Autodesk Inventor part; units mm, degrees
ref_plane "Work Plane1" through (99.0561, 66.015, -1.0424) normal (0, 1, 0) x (-0.9985, 0, 0.0543)
ref_plane "YZ Plane" through (0, 0, 0) normal (1, 0, 0) x (0, 1, 0)
ref_plane "XZ Plane" through (0, 0, 0) normal (0, 1, 0) x (-1, 0, 0)
ref_plane "Work Plane1" through (99.0561, 66.015, -1.0424) normal (0, 1, 0) x (-0.9985, 0, 0.0543)
sketch "Sketch1" plane through (99.0561, 66.015, -1.0424) normal (0, 1, 0) x (-0.9985, 0, 0.0543)
  circle A0 centre (-73.639, 4.9709) radius 7.75
  arc A1 (-74.285, 11.1523) -> (-74.9346, 11.0494) centre (-73.639, 4.9709) ccw
  line L0 (-74.039, 10.5582) -> (-74.285, 11.1523)
  line L1 (-73.239, 10.5582) -> (-74.039, 10.5582)
  line L2 (-72.9929, 11.1523) -> (-73.239, 10.5582)
  arc A2 (-72.3433, 11.0494) -> (-72.9929, 11.1523) centre (-73.639, 4.9709) ccw
  line L3 (-72.2928, 10.4083) -> (-72.3433, 11.0494)
  line L4 (-71.532, 10.1611) -> (-72.2928, 10.4083)
  line L5 (-71.1144, 10.6501) -> (-71.532, 10.1611)
  arc A3 (-70.5284, 10.3515) -> (-71.1144, 10.6501) centre (-73.639, 4.9709) ccw
  line L6 (-70.6785, 9.7262) -> (-70.5284, 10.3515)
  line L7 (-70.0313, 9.256) -> (-70.6785, 9.7262)
  line L8 (-69.483, 9.592) -> (-70.0313, 9.256)
  arc A4 (-69.0179, 9.1269) -> (-69.483, 9.592) centre (-73.639, 4.9709) ccw
  line L9 (-69.3539, 8.5786) -> (-69.0179, 9.1269)
  line L10 (-68.8837, 7.9314) -> (-69.3539, 8.5786)
  line L11 (-68.2584, 8.0815) -> (-68.8837, 7.9314)
  arc A5 (-67.9598, 7.4955) -> (-68.2584, 8.0815) centre (-73.639, 4.9709) ccw
  line L12 (-68.4488, 7.0779) -> (-67.9598, 7.4955)
  line L13 (-68.2016, 6.3171) -> (-68.4488, 7.0779)
  line L14 (-67.5605, 6.2666) -> (-68.2016, 6.3171)
  arc A6 (-67.4576, 5.617) -> (-67.5605, 6.2666) centre (-73.639, 4.9709) ccw
  line L15 (-68.0517, 5.3709) -> (-67.4576, 5.617)
  line L16 (-68.0517, 4.5709) -> (-68.0517, 5.3709)
  line L17 (-67.4576, 4.3249) -> (-68.0517, 4.5709)
  arc A7 (-67.5605, 3.6753) -> (-67.4576, 4.3249) centre (-73.639, 4.9709) ccw
  line L18 (-68.2016, 3.6248) -> (-67.5605, 3.6753)
  line L19 (-68.4488, 2.864) -> (-68.2016, 3.6248)
  line L20 (-67.9598, 2.4463) -> (-68.4488, 2.864)
  arc A8 (-68.2584, 1.8603) -> (-67.9598, 2.4463) centre (-73.639, 4.9709) ccw
  line L21 (-68.8837, 2.0105) -> (-68.2584, 1.8603)
  line L22 (-69.3539, 1.3632) -> (-68.8837, 2.0105)
  line L23 (-69.0179, 0.815) -> (-69.3539, 1.3632)
  arc A9 (-69.483, 0.3499) -> (-69.0179, 0.815) centre (-73.639, 4.9709) ccw
  line L24 (-70.0313, 0.6859) -> (-69.483, 0.3499)
  line L25 (-70.6785, 0.2157) -> (-70.0313, 0.6859)
  line L26 (-70.5284, -0.4096) -> (-70.6785, 0.2157)
  arc A10 (-71.1144, -0.7082) -> (-70.5284, -0.4096) centre (-73.639, 4.9709) ccw
  line L27 (-71.532, -0.2192) -> (-71.1144, -0.7082)
  line L28 (-72.2928, -0.4664) -> (-71.532, -0.2192)
  line L29 (-72.3433, -1.1075) -> (-72.2928, -0.4664)
  arc A11 (-72.9929, -1.2104) -> (-72.3433, -1.1075) centre (-73.639, 4.9709) ccw
  line L30 (-73.239, -0.6163) -> (-72.9929, -1.2104)
  line L31 (-74.039, -0.6163) -> (-73.239, -0.6163)
  line L32 (-74.285, -1.2104) -> (-74.039, -0.6163)
  arc A12 (-74.9346, -1.1075) -> (-74.285, -1.2104) centre (-73.639, 4.9709) ccw
  line L33 (-74.9851, -0.4664) -> (-74.9346, -1.1075)
  line L34 (-75.7459, -0.2192) -> (-74.9851, -0.4664)
  line L35 (-76.1636, -0.7082) -> (-75.7459, -0.2192)
  arc A13 (-76.7496, -0.4096) -> (-76.1636, -0.7082) centre (-73.639, 4.9709) ccw
  line L36 (-76.5994, 0.2157) -> (-76.7496, -0.4096)
  line L37 (-77.2467, 0.6859) -> (-76.5994, 0.2157)
  line L38 (-77.7949, 0.3499) -> (-77.2467, 0.6859)
  arc A14 (-78.26, 0.815) -> (-77.7949, 0.3499) centre (-73.639, 4.9709) ccw
  line L39 (-77.924, 1.3632) -> (-78.26, 0.815)
  line L40 (-78.3942, 2.0105) -> (-77.924, 1.3632)
  line L41 (-79.0195, 1.8603) -> (-78.3942, 2.0105)
  arc A15 (-79.3181, 2.4463) -> (-79.0195, 1.8603) centre (-73.639, 4.9709) ccw
  line L42 (-78.8291, 2.864) -> (-79.3181, 2.4463)
  line L43 (-79.0763, 3.6248) -> (-78.8291, 2.864)
  line L44 (-79.7174, 3.6753) -> (-79.0763, 3.6248)
  arc A16 (-79.8203, 4.3249) -> (-79.7174, 3.6753) centre (-73.639, 4.9709) ccw
  line L45 (-79.2262, 4.5709) -> (-79.8203, 4.3249)
  line L46 (-79.2262, 5.3709) -> (-79.2262, 4.5709)
  line L47 (-79.8203, 5.617) -> (-79.2262, 5.3709)
  arc A17 (-79.7174, 6.2666) -> (-79.8203, 5.617) centre (-73.639, 4.9709) ccw
  line L48 (-79.0763, 6.3171) -> (-79.7174, 6.2666)
  line L49 (-78.8291, 7.0779) -> (-79.0763, 6.3171)
  line L50 (-79.3181, 7.4955) -> (-78.8291, 7.0779)
  arc A18 (-79.0195, 8.0815) -> (-79.3181, 7.4955) centre (-73.639, 4.9709) ccw
  line L51 (-78.3942, 7.9314) -> (-79.0195, 8.0815)
  line L52 (-77.924, 8.5786) -> (-78.3942, 7.9314)
  line L53 (-78.26, 9.1269) -> (-77.924, 8.5786)
  arc A19 (-77.7949, 9.592) -> (-78.26, 9.1269) centre (-73.639, 4.9709) ccw
  line L54 (-77.2467, 9.256) -> (-77.7949, 9.592)
  line L55 (-76.5994, 9.7262) -> (-77.2467, 9.256)
  line L56 (-76.7496, 10.3515) -> (-76.5994, 9.7262)
  arc A20 (-76.1636, 10.6501) -> (-76.7496, 10.3515) centre (-73.639, 4.9709) ccw
  line L57 (-75.7459, 10.1611) -> (-76.1636, 10.6501)
  line L58 (-74.9851, 10.4083) -> (-75.7459, 10.1611)
  line L59 (-74.9346, 11.0494) -> (-74.9851, 10.4083)
  circle A21 centre (76.3213, 1.5167) radius 8.5
  arc A22 (76.017, 7.7243) -> (75.3526, 7.6558) centre (76.3213, 1.5167) ccw
  line L60 (76.226, 7.1302) -> (76.017, 7.7243)
  line L61 (77.0249, 7.0867) -> (76.226, 7.1302)
  line L62 (77.2971, 7.6546) -> (77.0249, 7.0867)
  arc A23 (77.9501, 7.5145) -> (77.2971, 7.6546) centre (76.3213, 1.5167) ccw
  line L63 (77.9654, 6.8849) -> (77.9501, 7.5145)
  line L64 (78.7116, 6.5967) -> (77.9654, 6.8849)
  line L65 (79.1461, 7.0527) -> (78.7116, 6.5967)
  arc A24 (79.7238, 6.7176) -> (79.1461, 7.0527) centre (76.3213, 1.5167) ccw
  line L66 (79.5437, 6.1141) -> (79.7238, 6.7176)
  line L67 (80.1645, 5.6094) -> (79.5437, 6.1141)
  line L68 (80.7185, 5.9088) -> (80.1645, 5.6094)
  arc A25 (81.1644, 5.4116) -> (80.7185, 5.9088) centre (76.3213, 1.5167) ccw
  line L69 (80.8067, 4.8933) -> (81.1644, 5.4116)
  line L70 (81.2411, 4.2215) -> (80.8067, 4.8933)
  line L71 (81.8605, 4.335) -> (81.2411, 4.2215)
  arc A26 (82.131, 3.7243) -> (81.8605, 4.335) centre (76.3213, 1.5167) ccw
  line L72 (81.6306, 3.3419) -> (82.131, 3.7243)
  line L73 (81.8361, 2.5688) -> (81.6306, 3.3419)
  line L74 (82.4603, 2.4853) -> (81.8361, 2.5688)
  arc A27 (82.5288, 1.821) -> (82.4603, 2.4853) centre (76.3213, 1.5167) ccw
  line L75 (81.9347, 1.6119) -> (82.5288, 1.821)
  line L76 (81.8913, 0.8131) -> (81.9347, 1.6119)
  line L77 (82.4592, 0.5409) -> (81.8913, 0.8131)
  arc A28 (82.319, -0.1121) -> (82.4592, 0.5409) centre (76.3213, 1.5167) ccw
  line L78 (81.6894, -0.1274) -> (82.319, -0.1121)
  line L79 (81.4012, -0.8737) -> (81.6894, -0.1274)
  line L80 (81.8572, -1.3081) -> (81.4012, -0.8737)
  arc A29 (81.5221, -1.8858) -> (81.8572, -1.3081) centre (76.3213, 1.5167) ccw
  line L81 (80.9186, -1.7058) -> (81.5221, -1.8858)
  line L82 (80.4139, -2.3265) -> (80.9186, -1.7058)
  line L83 (80.7133, -2.8805) -> (80.4139, -2.3265)
  arc A30 (80.2161, -3.3264) -> (80.7133, -2.8805) centre (76.3213, 1.5167) ccw
  line L84 (79.6978, -2.9687) -> (80.2161, -3.3264)
  line L85 (79.026, -3.4031) -> (79.6978, -2.9687)
  line L86 (79.1395, -4.0225) -> (79.026, -3.4031)
  arc A31 (78.5289, -4.293) -> (79.1395, -4.0225) centre (76.3213, 1.5167) ccw
  line L87 (78.1465, -3.7926) -> (78.5289, -4.293)
  line L88 (77.3733, -3.9981) -> (78.1465, -3.7926)
  line L89 (77.2899, -4.6223) -> (77.3733, -3.9981)
  arc A32 (76.6255, -4.6908) -> (77.2899, -4.6223) centre (76.3213, 1.5167) ccw
  line L90 (76.4165, -4.0967) -> (76.6255, -4.6908)
  line L91 (75.6177, -4.0533) -> (76.4165, -4.0967)
  line L92 (75.3454, -4.6212) -> (75.6177, -4.0533)
  arc A33 (74.6924, -4.481) -> (75.3454, -4.6212) centre (76.3213, 1.5167) ccw
  line L93 (74.6772, -3.8514) -> (74.6924, -4.481)
  line L94 (73.9309, -3.5632) -> (74.6772, -3.8514)
  line L95 (73.4964, -4.0192) -> (73.9309, -3.5632)
  arc A34 (72.9187, -3.6841) -> (73.4964, -4.0192) centre (76.3213, 1.5167) ccw
  line L96 (73.0988, -3.0806) -> (72.9187, -3.6841)
  line L97 (72.4781, -2.5759) -> (73.0988, -3.0806)
  line L98 (71.924, -2.8754) -> (72.4781, -2.5759)
  arc A35 (71.4781, -2.3781) -> (71.924, -2.8754) centre (76.3213, 1.5167) ccw
  line L99 (71.8358, -1.8598) -> (71.4781, -2.3781)
  line L100 (71.4015, -1.188) -> (71.8358, -1.8598)
  line L101 (70.782, -1.3016) -> (71.4015, -1.188)
  arc A36 (70.5116, -0.6909) -> (70.782, -1.3016) centre (76.3213, 1.5167) ccw
  line L102 (71.012, -0.3085) -> (70.5116, -0.6909)
  line L103 (70.8064, 0.4647) -> (71.012, -0.3085)
  line L104 (70.1822, 0.5481) -> (70.8064, 0.4647)
  arc A37 (70.1137, 1.2125) -> (70.1822, 0.5481) centre (76.3213, 1.5167) ccw
  line L105 (70.7078, 1.4215) -> (70.1137, 1.2125)
  line L106 (70.7513, 2.2203) -> (70.7078, 1.4215)
  line L107 (70.1834, 2.4926) -> (70.7513, 2.2203)
  arc A38 (70.3235, 3.1456) -> (70.1834, 2.4926) centre (76.3213, 1.5167) ccw
  line L108 (70.9531, 3.1608) -> (70.3235, 3.1456)
  line L109 (71.2413, 3.9071) -> (70.9531, 3.1608)
  line L110 (70.7853, 4.3415) -> (71.2413, 3.9071)
  arc A39 (71.1204, 4.9193) -> (70.7853, 4.3415) centre (76.3213, 1.5167) ccw
  line L111 (71.7239, 4.7392) -> (71.1204, 4.9193)
  line L112 (72.2286, 5.3599) -> (71.7239, 4.7392)
  line L113 (71.9292, 5.914) -> (72.2286, 5.3599)
  arc A40 (72.4264, 6.3599) -> (71.9292, 5.914) centre (76.3213, 1.5167) ccw
  line L114 (72.9447, 6.0021) -> (72.4264, 6.3599)
  line L115 (73.6165, 6.4365) -> (72.9447, 6.0021)
  line L116 (73.503, 7.056) -> (73.6165, 6.4365)
  arc A41 (74.1136, 7.3264) -> (73.503, 7.056) centre (76.3213, 1.5167) ccw
  line L117 (74.496, 6.826) -> (74.1136, 7.3264)
  line L118 (75.2692, 7.0315) -> (74.496, 6.826)
  line L119 (75.3526, 7.6558) -> (75.2692, 7.0315)
  line L120 (76.1551, -5.6964) -> (-73.8051, -2.2421)
  line L121 (76.4874, 8.7298) -> (-73.4728, 12.184)
  arc A42 (76.1551, -5.6964) -> (76.4874, 8.7298) centre (76.3213, 1.5167) ccw
  arc A43 (-73.4958, 11.1843) -> (-73.7821, -1.2424) centre (-73.639, 4.9709) ccw
  arc A44 (-73.4728, 12.184) -> (-73.8051, -2.2421) centre (-73.639, 4.9709) ccw
  line L122 (-73.7821, -1.2424) -> (76.1781, -4.6966)
  arc A45 (76.1781, -4.6966) -> (76.017, 7.7243) centre (76.3213, 1.5167) ccw
  line L123 (76.4644, 7.7301) -> (-73.4958, 11.1843)
  point P0 (98.9665, -4.3398)
  dimension "d1" = 1
  dimension "d2" = 1
extrude "Extrusion1" add sketch "Sketch1" along normal blind 6 contours L123 A43 A1 A20 A19 A18 A17 A16 A15 A14 A13 A12 L122 A0 L120 A44 L121 | A0 L121 A21 L123 | L122 A21 L120 A0 | A21 L121 A42 L120 L122 A45 A32 A31 A30 A29 A28 A27 A26 A25 A24 A23 L123
properties part number "Tandrem"
Can you work these out from the model? Positions are in its coordinate system, mm. Give positions to 0.01 mm unless a question says otherwise; leave off trailing zeros. Loops run counter-clockwise (first coordinate to the right, second up) from the corner with the lowest first, then second, coordinate; pieces in that order, holes last. Notation, with made-up numbers: (89.5, -2) - (143.5, -2) arc R29 cw to (143.5, 30) - close; hole circle Ø6 at (31.5, 33). An arc over 180 degrees is marked (long way). One line per item, written item: value.
(1) If we section it at B-B, the plane x = 130.5: List the corners of the cut face in (y, z) for me (3 decimals).
Verdict:
outline: (66.015, -5.97) - (72.015, -5.97) - (72.015, -4.969) - (66.015, -4.969) - close; (66.015, 7.467) - (72.015, 7.467) - (72.015, 8.467) - (66.015, 8.467) - close
(2) If we section it at A-A, the plane x = 166: List the corners of the cut face in (y, z) for me (3 decimals), plus the area to 3 significant figures.
Verdict:
outline: (66.015, -7.081) - (72.015, -7.081) - (72.015, -6.081) - (66.015, -6.081) - close; (66.015, 6.355) - (72.015, 6.355) - (72.015, 7.356) - (66.015, 7.356) - close
area: 12.0 mm^2
(3) I need wall thicknesses on line 1 along Z through (x, y) = (27, 70.35); line 2 along Z through (x, y) = (118.5, 67.5); line 3 along X through (y, z) = (67.95, 2.75). Which ranges of each line are inside material? Lowest first, please.
Verdict:
line 1: -2.73 to -1.73, 10.71 to 11.71
line 2: -5.59 to -4.59, 7.84 to 8.84
line 3: 15.96 to 17, 178.39 to 179.49
(4) I'm going to push a flat-ended pin straight in: pin 1 (3 mm diameter, centred on y = 70, z = 8, fed in from -X). Where does the tip first touch, or does it pass through?
Verdict:
pin 1: x = 15.96
